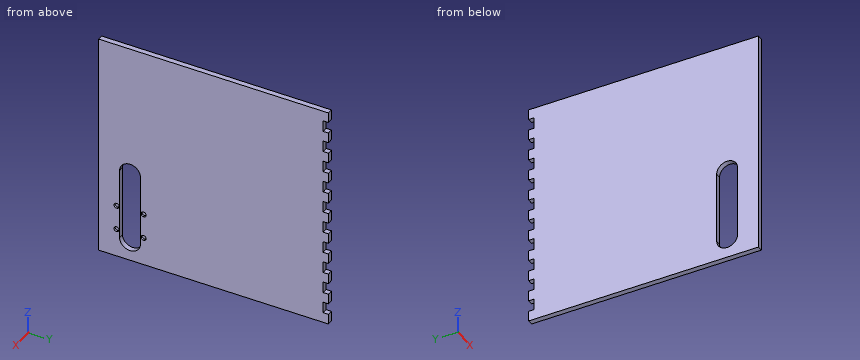
from build123d import *

# Parameters (mm, degrees)
SKETCH1_W           = 279.4
SKETCH1_H           = 285.75
BOSS_EXTRUDE1_DEPTH = 6.35
SKETCH2_W           = 279.4
SKETCH2_H           = 6.35
BOSS_EXTRUDE2_DEPTH = 12.7
CUT_EXTRUDE1_DEPTH  = 20.05
SKETCH5_W           = 51.415141408
SKETCH5_H           = 21.159166417
CUT_EXTRUDE2_DEPTH  = 280.4
SKETCH4_W           = 13.97
SKETCH4_H           = 6.35
CUT_EXTRUDE3_DEPTH  = 6.35
CUT_EXTRUDE5_DEPTH  = 2.54
SKETCH7_W           = 279.4
SKETCH7_H           = 6.35
CUT_EXTRUDE6_DEPTH  = 7.35


with BuildPart() as part:
    # Sketch1 → Boss-Extrude1 (new body)
    with BuildSketch(Plane(origin=(0, 0, 0), x_dir=(0, 0, -1), z_dir=(1, 0, 0))):
        Rectangle(SKETCH1_W, SKETCH1_H)
    extrude(amount=BOSS_EXTRUDE1_DEPTH)

    # Sketch2 → Boss-Extrude2 (add)
    with BuildSketch(Plane(origin=(6.35, 0, 0), x_dir=(0, 0, -1), z_dir=(1, 0, 0))):
        with Locations((0, 139.7)):
            Rectangle(SKETCH2_W, SKETCH2_H)
    extrude(amount=BOSS_EXTRUDE2_DEPTH)

    # Sketch3 → Cut-Extrude1 (cut, through all)
    with BuildSketch(Plane.ZY):
        with BuildLine():
            Line((-114.3, -85.725), (-25.4, -85.725))
            ThreePointArc((-25.4, -85.725), (-12.7, -98.425), (-25.4, -111.125))
            Line((-25.4, -111.125), (-114.3, -111.125))
            ThreePointArc((-114.3, -111.125), (-127, -98.425), (-114.3, -85.725))
        make_face()
    extrude(amount=-CUT_EXTRUDE1_DEPTH, mode=Mode.SUBTRACT)

    # Sketch5 → Cut-Extrude2 (cut, through all)
    with BuildSketch(Plane(origin=(0, 0, -139.7), x_dir=(-1, 0, 0), z_dir=(0, 0, -1))):
        with Locations((-32.057570704, 147.104583209)):
            Rectangle(SKETCH5_W, SKETCH5_H)
    extrude(amount=-CUT_EXTRUDE2_DEPTH, mode=Mode.SUBTRACT)

    # Sketch4 → Cut-Extrude3 (cut)
    with BuildSketch(Plane.ZY):
        with Locations((-120.015, 139.7)):
            Rectangle(SKETCH4_W, SKETCH4_H)
        with Locations((-93.345, 139.7)):
            Rectangle(SKETCH4_W, SKETCH4_H)
        with Locations((-66.675, 139.7)):
            Rectangle(SKETCH4_W, SKETCH4_H)
        with Locations((-40.005, 139.7)):
            Rectangle(SKETCH4_W, SKETCH4_H)
        with Locations((-13.335, 139.7)):
            Rectangle(SKETCH4_W, SKETCH4_H)
        with Locations((13.335, 139.7)):
            Rectangle(SKETCH4_W, SKETCH4_H)
        with Locations((40.005, 139.7)):
            Rectangle(SKETCH4_W, SKETCH4_H)
        with Locations((66.675, 139.7)):
            Rectangle(SKETCH4_W, SKETCH4_H)
        with Locations((93.345, 139.7)):
            Rectangle(SKETCH4_W, SKETCH4_H)
        with Locations((120.015, 139.7)):
            Rectangle(SKETCH4_W, SKETCH4_H)
    extrude(amount=-CUT_EXTRUDE3_DEPTH, mode=Mode.SUBTRACT)

    # Sketch6 → Cut-Extrude5 (cut)
    with BuildSketch(Plane(origin=(6.35, 0, 0), x_dir=(0, 0, -1), z_dir=(1, 0, 0))):
        with BuildLine():
            ThreePointArc((76.575, -82.06), (75.64506403, -79.81493597), (73.4, -78.885))
            ThreePointArc((73.4, -78.885), (74.460660172, -79.324339828), (74.9, -80.385))
            Line((74.9, -80.385), (74.9, -84.858325392))
            ThreePointArc((74.9, -84.858325392), (76.124254485, -83.690663209), (76.575, -82.06))
        make_face()
        with BuildLine():
            Line((71.9, -80.385), (71.9, -84.858325392))
            ThreePointArc((71.9, -84.858325392), (73.4, -85.235), (74.9, -84.858325392))
            Line((74.9, -84.858325392), (74.9, -80.385))
            ThreePointArc((74.9, -80.385), (74.460660172, -79.324339828), (73.4, -78.885))
            ThreePointArc((73.4, -78.885), (72.339339828, -79.324339828), (71.9, -80.385))
        make_face()
        with BuildLine():
            ThreePointArc((73.4, -78.885), (70.320608167, -81.286714193), (71.9, -84.858325392))
            Line((71.9, -84.858325392), (71.9, -80.385))
            ThreePointArc((71.9, -80.385), (72.339339828, -79.324339828), (73.4, -78.885))
        make_face()
        with BuildLine():
            Line((102.9, -80.385), (102.9, -84.858325392))
            ThreePointArc((102.9, -84.858325392), (104.4, -85.235), (105.9, -84.858325392))
            Line((105.9, -84.858325392), (105.9, -80.385))
            ThreePointArc((105.9, -80.385), (105.460660172, -79.324339828), (104.4, -78.885))
            ThreePointArc((104.4, -78.885), (103.339339828, -79.324339828), (102.9, -80.385))
        make_face()
        with BuildLine():
            ThreePointArc((104.4, -78.885), (101.320608167, -81.286714193), (102.9, -84.858325392))
            Line((102.9, -84.858325392), (102.9, -80.385))
            ThreePointArc((102.9, -80.385), (103.339339828, -79.324339828), (104.4, -78.885))
        make_face()
        with BuildLine():
            ThreePointArc((107.575, -82.06), (106.64506403, -79.81493597), (104.4, -78.885))
            ThreePointArc((104.4, -78.885), (105.460660172, -79.324339828), (105.9, -80.385))
            Line((105.9, -80.385), (105.9, -84.858325392))
            ThreePointArc((105.9, -84.858325392), (107.124254485, -83.690663209), (107.575, -82.06))
        make_face()
        with BuildLine():
            ThreePointArc((74.9, -116.465), (74.460660172, -117.525660172), (73.4, -117.965))
            ThreePointArc((73.4, -117.965), (75.64506403, -117.03506403), (76.575, -114.79))
            ThreePointArc((76.575, -114.79), (76.124254485, -113.159336791), (74.9, -111.991674608))
            Line((74.9, -111.991674608), (74.9, -116.465))
        make_face()
        with BuildLine():
            Line((71.9, -111.991674608), (71.9, -116.465))
            ThreePointArc((71.9, -116.465), (72.339339828, -117.525660172), (73.4, -117.965))
            ThreePointArc((73.4, -117.965), (74.460660172, -117.525660172), (74.9, -116.465))
            Line((74.9, -116.465), (74.9, -111.991674608))
            ThreePointArc((74.9, -111.991674608), (73.4, -111.615), (71.9, -111.991674608))
        make_face()
        with BuildLine():
            ThreePointArc((73.4, -117.965), (72.339339828, -117.525660172), (71.9, -116.465))
            Line((71.9, -116.465), (71.9, -111.991674608))
            ThreePointArc((71.9, -111.991674608), (70.320608167, -115.563285807), (73.4, -117.965))
        make_face()
        with BuildLine():
            ThreePointArc((104.4, -117.965), (105.460660172, -117.525660172), (105.9, -116.465))
            Line((105.9, -116.465), (105.9, -111.991674608))
            ThreePointArc((105.9, -111.991674608), (104.4, -111.615), (102.9, -111.991674608))
            Line((102.9, -111.991674608), (102.9, -116.465))
            ThreePointArc((102.9, -116.465), (103.339339828, -117.525660172), (104.4, -117.965))
        make_face()
        with BuildLine():
            Line((105.9, -111.991674608), (105.9, -116.465))
            ThreePointArc((105.9, -116.465), (105.460660172, -117.525660172), (104.4, -117.965))
            ThreePointArc((104.4, -117.965), (106.64506403, -117.03506403), (107.575, -114.79))
            ThreePointArc((107.575, -114.79), (107.124254485, -113.159336791), (105.9, -111.991674608))
        make_face()
        with BuildLine():
            ThreePointArc((102.9, -111.991674608), (101.320608167, -115.563285807), (104.4, -117.965))
            ThreePointArc((104.4, -117.965), (103.339339828, -117.525660172), (102.9, -116.465))
            Line((102.9, -116.465), (102.9, -111.991674608))
        make_face()
    extrude(amount=-CUT_EXTRUDE5_DEPTH, mode=Mode.SUBTRACT)

    # Sketch7 → Cut-Extrude6 (cut, through all)
    with BuildSketch(Plane(origin=(6.35, 0, 0), x_dir=(0, 0, -1), z_dir=(1, 0, 0))):
        with Locations((0, -139.7)):
            Rectangle(SKETCH7_W, SKETCH7_H)
    extrude(amount=-CUT_EXTRUDE6_DEPTH, mode=Mode.SUBTRACT)


solid = part.part
The listing builds one solid part. Answer for the finished solid, in the listing's coordinates (mm). Coordinates: 2 decimals unless noted, no trailing zeros.
Q1. Consider line 1 (Y direction, x = 1, z = -49.5) (3 decimals); line 2 (Y direction, x = 5, z = -74.5) (3 decimals); line 3 (Z direction, x = 5.25, y = -113.5). Determine where each line is inside the solid, lowest interval first.
Q2. Given P1, Ø3, axis at x = 2.5, z = 37.5, coming from the +Y side (3 decimals); P2, Ø1.9, axis at y = -115.5, z = -74.5, coming from the +X side, each flat-ended and moving along its own axis, determine where each tip first touches the part or whether it passes through.
Q3. A cutting plane is placed at A-A, the plane x = 5. State how many separate pieces and enclosed holes the cut face has, and give its area (3 significant figures).
Answers follow:
1. line 1: y = -136.525 to -111.125, -85.725 to 142.875
1. line 2: y = -136.525 to -117.768, -111.812 to -111.125, -85.725 to -85.038, -79.082 to 142.875
1. line 3: z = -139.7 to -107.3, -101.5 to -76.3, -70.5 to 139.7
2. P1: stops at y = 136.525
2. P2: stops at x = 3.81
3. separate pieces: 1
3. enclosed holes: 5
3. area: 74,300 mm2
